```python
from build123d import *

# Parameters (mm, degrees)
F1_DEPTH = 12.7


with BuildPart() as f1:
    # F0 (on Top) → F1 (new body)
    with BuildSketch(Plane.XY):
        with BuildLine():
            ThreePointArc((-14.433566, 29.576561), (-14.026399, 30.402215), (-13.168399, 30.735873))
            Line((-13.168399, 30.735873), (13.96812, 30.735873))
            ThreePointArc((13.96812, 30.735873), (14.826119, 30.402215), (15.233287, 29.576561))
            Line((15.233287, 29.576561), (21.672975, -44.029412))
            ThreePointArc((21.672975, -44.029412), (22.011711, -44.787415), (22.74638, -45.174163))
            Line((22.74638, -45.174163), (24.260408, -45.174163))
            ThreePointArc((24.260408, -45.174163), (25.176504, -44.783746), (25.529358, -43.852536))
            Line((25.529358, -43.852536), (23.274442, 11.57156))
            Line((23.274442, 11.57156), (30.972435, 13.634231))
            Line((30.972435, 13.634231), (32.855034, 14.138672))
            ThreePointArc((32.855034, 14.138672), (33.533893, 14.592271), (33.796334, 15.365398))
            Line((33.796334, 15.365398), (28.913047, 33.590075))
            ThreePointArc((28.913047, 33.590075), (28.459448, 34.268934), (27.686321, 34.531375))
            Line((27.686321, 34.531375), (26.37152, 34.531375))
            ThreePointArc((26.37152, 34.531375), (25.363961, 34.034502), (25.144794, 32.932675))
            Line((25.144794, 32.932675), (29.371674, 17.157746))
            Line((29.371674, 17.157746), (23.115372, 15.481375))
            Line((23.115372, 15.481375), (18.26316, 33.590075))
            ThreePointArc((18.26316, 33.590075), (17.809562, 34.268934), (17.036435, 34.531375))
            Line((17.036435, 34.531375), (-17.021739, 34.531375))
            ThreePointArc((-17.021739, 34.531375), (-17.881974, 34.195664), (-18.287421, 33.366013))
            Line((-18.287421, 33.366013), (-24.668649, -43.820158))
            ThreePointArc((-24.668649, -43.820158), (-24.333586, -44.788999), (-23.392157, -45.19475))
            Line((-23.392157, -45.19475), (-22.127202, -45.183983))
            ThreePointArc((-22.127202, -45.183983), (-21.276035, -44.846712), (-20.872844, -44.024717))
            Line((-20.872844, -44.024717), (-14.433566, 29.576561))
        make_face()
    extrude(amount=F1_DEPTH)


solid = f1.part
```
Can you work these out from the model? Positions are in its coordinate system, mm. A direction names the side the tool comes from. Round coordinates to 2 decimals unless told otherwise and drop trailing zeros. Loops run counter-clockwise (first coordinate to the right, second up) from the corner with the lowest first, then second, coordinate; pieces in that order, holes last.
Item 1: Suppose I cut it at D-D, the plane x = 7. Write out the boundary of the cut face in (y, z).
Item 2: Suppose I cut it at A-A, the plane y = 3.5. Write out the boundary of the cut face in (x, z), then the cut area to 3 significant figures.
Item 3: Please list where these lines run through material, in increasing order: L1, parallel to Y at x = 7, z = 5.5; L2, parallel to X at y = 6, z = 11; L3, parallel to X at y = 11, z = 11.5.
Item 4: Will these pins go through, and if not, where does the flat tip stop? pin 1 Ø5 at (y, z) = (-29, 4.5) entering from -X; pin 2 Ø6.5 at (x, z) = (-1.5, 8.5) entering from -Y; pin 3 Ø0.5 at (x, z) = (23.5, 9) entering from -Y.
Item 5: If we mould it in two halves opening along X, with no side actions, what happens to faces 5 (the flat face through (18.408, -6.711, 6.261)), 6 (the flat face through (0, 34.531, 6)), 7 (the flat face through (-21.433, -4.687, 6.261))? For each: +X half, -X half, draft (parallel to the pull), parting line (faces both ways), or undercut.
Item 6: Suppose I cut it at C-C, the plane y = 27. Write out the boundary of the cut face in (x, z).
Item 7: Suppose I cut it at B-B, the plane z = 9. Write out the boundary of the cut face in (x, y).
Item 8: Which directions (+Z, -Z, +X, -X, +Y, -Y) give clear straight access to the entire face, cutting with the end or side of a thin tool? Please do faces 1 (the flat face through (26.29, 16.33, 6.26)), 2 (the flat face through (-17.7, -7.74, 6.26)), 3 (the flat face through (24.418, -16.528, 6.261)), 4 (the flat face through (20.723, 24.409, 6.261)).
Reported:
1. outline: (30.74, 0) - (34.53, 0) - (34.53, 12.7) - (30.74, 12.7) - close
2. outline: (-20.76, 0) - (-16.71, 0) - (-16.71, 12.7) - (-20.76, 12.7) - close; (17.51, 0) - (23.6, 0) - (23.6, 12.7) - (17.51, 12.7) - close
2. area: 129 mm2
3. L1: y = 30.74 to 34.53
3. L2: x = -20.55 to -16.5, 17.3 to 23.5
3. L3: x = -20.14 to -16.06, 16.86 to 23.3
4. pin 1: stops at x = -23.65
4. pin 2: stops at y = 30.74
4. pin 3: stops at y = -45.17
5. face 5: undercut
5. face 6: draft
5. face 7: -X half
6. outline: (-18.81, 0) - (-14.66, 0) - (-14.66, 12.7) - (-18.81, 12.7) - close; (15.46, 0) - (20.03, 0) - (20.03, 12.7) - (15.46, 12.7) - close; (26.73, 0) - (30.68, 0) - (30.68, 12.7) - (26.73, 12.7) - close
7. outline: (-24.67, -43.82) arc R1.27 ccw to (-23.39, -45.19) - (-22.13, -45.18) arc R1.27 ccw to (-20.87, -44.02) - (-14.43, 29.58) arc R1.27 cw to (-13.17, 30.74) - (13.97, 30.74) arc R1.27 cw to (15.23, 29.58) - (21.67, -44.03) arc R1.27 ccw to (22.75, -45.17) - (24.26, -45.17) arc R1.27 ccw to (25.53, -43.85) - (23.27, 11.57) - (32.86, 14.14) arc R1.27 ccw to (33.8, 15.37) - (28.91, 33.59) arc R1.27 ccw to (27.69, 34.53) - (26.37, 34.53) arc R1.27 ccw to (25.14, 32.93) - (29.37, 17.16) - (23.12, 15.48) - (18.26, 33.59) arc R1.27 ccw to (17.04, 34.53) - (-17.02, 34.53) arc R1.27 ccw to (-18.29, 33.37) - close
8. face 1: +Z, -Z
8. face 2: +Z, -Z, -Y
8. face 3: +Z, -Z, +X
8. face 4: +Z, -Z, +Y
